from build123d import *

# Parameters (mm, degrees)
BOSS_EXTRUDE1_DEPTH = 50
CHAMFER1_SIZE       = 5
SKETCH2_R           = 1.625
SKETCH2_R_2         = 12.5
CUT_EXTRUDE1_DEPTH  = 77.681158051
CUT_EXTRUDE2_DEPTH  = 89.971905678
BOSS_EXTRUDE2_DEPTH = 1
BOSS_EXTRUDE3_START = -50
BOSS_EXTRUDE3_DEPTH = 1


with BuildPart() as part:
    # Sketch1 → Boss-Extrude1 (new body)
    with BuildSketch(Plane(origin=(0, 0, 0), x_dir=(0, 0, -1), z_dir=(1, 0, 0))):
        Polygon((-26, 0), (26, 0), (26, 54), (24, 54), (24, 2), (-26, 2), align=None)
    extrude(amount=-BOSS_EXTRUDE1_DEPTH)

    # Chamfer1
    chamfer1_edges = [part.edges().sort_by_distance(p)[0] for p in [
        (-50, 54, -25),
        (-50, 1, 26),
        (0, 54, -25),
        (0, 1, 26),
    ]]
    chamfer(chamfer1_edges, length=CHAMFER1_SIZE)

    # Sketch2 → Cut-Extrude1 (cut, through all)
    with BuildSketch(Plane(origin=(0, 2, 0), x_dir=(1, 0, 0), z_dir=(0, 1, 0))):
        with Locations(Location((-40.5, 13, 0), (0, 0, 270))):
            Circle(SKETCH2_R)
        with Locations(Location((-9.5, 13, 0), (0, 0, 90))):
            Circle(SKETCH2_R)
        with Locations(Location((-9.5, -18, 0), (0, 0, 270))):
            Circle(SKETCH2_R)
        with Locations(Location((-40.5, -18, 0), (0, 0, 90))):
            Circle(SKETCH2_R)
        with Locations(Location((-25, -2.5, 0), (0, 0, 270))):
            Circle(SKETCH2_R_2)
    extrude(amount=-CUT_EXTRUDE1_DEPTH, mode=Mode.SUBTRACT)

    # Sketch3 → Cut-Extrude2 (cut, through all)
    with BuildSketch(Plane.XY.offset(-24)):
        with BuildLine():
            Line((-38.5, 46), (-38.5, 10))
            ThreePointArc((-38.5, 10), (-40.5, 8), (-42.5, 10))
            Line((-42.5, 10), (-42.5, 46))
            ThreePointArc((-42.5, 46), (-40.5, 48), (-38.5, 46))
        make_face()
        with BuildLine():
            Line((-11.5, 46), (-11.5, 10))
            ThreePointArc((-11.5, 10), (-9.5, 8), (-7.5, 10))
            Line((-7.5, 10), (-7.5, 46))
            ThreePointArc((-7.5, 46), (-9.5, 48), (-11.5, 46))
        make_face()
    extrude(amount=-CUT_EXTRUDE2_DEPTH, mode=Mode.SUBTRACT)

    # Sketch4 → Boss-Extrude2 (add)
    with BuildSketch(Plane(origin=(0, 0, 0), x_dir=(0, 0, -1), z_dir=(1, 0, 0))):
        Polygon((9, 2), (24, 2), (24, 17), align=None)
    extrude(amount=-BOSS_EXTRUDE2_DEPTH)

    # Sketch4<2> → Boss-Extrude3 (add)
    with BuildSketch(Plane(origin=(0, 0, 0), x_dir=(0, 0, -1), z_dir=(1, 0, 0)).offset(BOSS_EXTRUDE3_START)):
        Polygon((9, 2), (24, 2), (24, 17), align=None)
    extrude(amount=BOSS_EXTRUDE3_DEPTH)


solid = part.part
The model under review builds one solid part; all positions refer to its coordinate system, in mm. A direction names the side the tool comes from. Coordinates: 2 decimals unless noted, no trailing zeros. Order: outer loops, then holes, each group sorted by start corner. A loop starts at its lowest first (then second) coordinate and runs counter-clockwise, first axis right, second up. Notation, with made-up numbers: (43, -30.5) -> (74, -30.5) arc R13 ccw to (74, -7.5) -> close; hole circle Ø6 at (-27, 10.5). An arc over 180 degrees is marked (long way). Answer in a Markdown table with one row per item.
(1) Consider section B-B (z = 10). Write out the cut boundary in (x, y).
Answers:
| item | result |
|---|---|
| outline | (-50, 0) -> (-35, 0) -> (-35, 2) -> (-50, 2) -> close; (-15, 0) -> (0, 0) -> (0, 2) -> (-15, 2) -> close |
(2) The part is to be moulded in two halves that separate along Z. For faces 4 (the cylindrical face through (-9.99, 1.01, -14.55)), 5 (the cylindrical face through (-37.203, 1.014, -0.21)), 6 (the flat face through (-25, 54, -25)), 7 (the flat face through (-25, 27, -26)), say which applies: +Z half, -Z half, draft (parallel to the pull), parting line (faces both ways), or undercut.
Answers:
| item | result |
|---|---|
| face 4 | undercut |
| face 5 | undercut |
| face 6 | draft |
| face 7 | -Z half |
(3) Wall thickness on line 1 along X through (y, z) = (0.8, 18) (3 decimals); line 2 along Z through (x, y) = (-4, 52); line 3 along Y through (x, z) = (-5, -5): over which ranges is each line inside the solid? List them lowest first.
Answers:
| item | result |
|---|---|
| line 1 | -50 to -42.125, -38.875 to -11.125, -7.875 to 0 |
| line 2 | -26 to -24 |
| line 3 | 0 to 2 |
(4) Consider section A-A (x = -25). Write out the cut boundary in (y, z).
Answers:
| item | result |
|---|---|
| outline | (0, -26) -> (54, -26) -> (54, -24) -> (2, -24) -> (2, -10) -> (0, -10) -> close; (0, 15) -> (2, 15) -> (2, 26) -> (0, 26) -> close |
(5) Machinability: for faces 1 (the flat face through (-0.5, 9.6, -16.6)), 2 (the flat face through (-25, 28, -24)), 3 (the cylindrical face through (-40.5, 8, -25)), which of the approach directions +Z, -Z, +X, -X, +Y, -Y give a long, thin tool a straight path to every point of the face, cutting with its end or side? Answer none if there is none.
Answers:
| item | result |
|---|---|
| face 1 | +Z, +X, -X, +Y |
| face 2 | +Z, +Y |
| face 3 | +Z, -Z |
(6) Consider section D-D (y = 13). Write out the cut boundary in (x, z).
Answers:
| item | result |
|---|---|
| outline | (-50, -26) -> (-42.5, -26) -> (-42.5, -24) -> (-49, -24) -> (-49, -20) -> (-50, -20) -> close; (-38.5, -26) -> (-11.5, -26) -> (-11.5, -24) -> (-38.5, -24) -> close; (-7.5, -26) -> (0, -26) -> (0, -20) -> (-1, -20) -> (-1, -24) -> (-7.5, -24) -> close |
(7) Insertion check: pin 1 (4 mm diameter, centred on x = -40.5, z = -13, fed in from +Y); pin 2 (15 mm diameter, centred on x = -24, y = 24.5, fed in from +Z); pin 3 (1.9 mm diameter, centred on x = -9.5, z = 18, fed in from -Y). Each pin has a flat end and moves straight along its axis. Give the tip position at first contact, or say it passes through.
Answers:
| item | result |
|---|---|
| pin 1 | y = 2 |
| pin 2 | z = -24 |
| pin 3 | through |
(8) Consider section C-C (z = -13). Write out the cut boundary in (x, y) (3 decimals).
Answers:
| item | result |
|---|---|
| outline | (-50, 0) -> (-42.125, 0) -> (-42.125, 2) -> (-49, 2) -> (-49, 6) -> (-50, 6) -> close; (-38.875, 0) -> (-11.125, 0) -> (-11.125, 2) -> (-38.875, 2) -> close; (-7.875, 0) -> (0, 0) -> (0, 6) -> (-1, 6) -> (-1, 2) -> (-7.875, 2) -> close |
